Design review of the part built by this model. Coordinates are the model's own, in mm. A direction names the side the tool comes from. Round coordinates to 2 decimals unless told otherwise and drop trailing zeros. Loops run counter-clockwise (first coordinate to the right, second up) from the corner with the lowest first, then second, coordinate; pieces in that order, holes last. Notation, with made-up numbers: (82, 28) -> (99, 28) arc R24 cw to (99, 48) -> close; hole circle Ø4 at (16.5, 84.25). An arc over 180 degrees is marked (long way). Use a Markdown table: item, result. Add a question column.
from build123d import *

# Parameters (mm, degrees)
ESBO_O1_W                       = 143.01
ESBO_O1_H                       = 101.6
RESSALTO_EXTRUS_O1_DEPTH        = 6.35
ESBO_O2_R                       = 2
CORTE_EXTRUS_O1_DEPTH           = 13
ESBO_O3_R                       = 2.6
CORTE_EXTRUS_O2_DEPTH           = 7
ESBO_O4_R                       = 4
CORTE_EXTRUS_O3_DEPTH           = 0.55
CROQUIS1_R                      = 4
CORTAR_EXTRUIR1_DEPTH           = 2
CORTAR_EXTRUIR1_DRAFT           = -45
CORTAR_EXTRUIR1_PROFILE_2_DEPTH = 2
CORTAR_EXTRUIR1_PROFILE_2_DRAFT = -45
CORTAR_EXTRUIR1_PROFILE_3_DEPTH = 2
CORTAR_EXTRUIR1_PROFILE_3_DRAFT = -45
CORTAR_EXTRUIR1_PROFILE_4_DEPTH = 2
CORTAR_EXTRUIR1_PROFILE_4_DRAFT = -45
CORTAR_EXTRUIR1_PROFILE_5_DEPTH = 2
CORTAR_EXTRUIR1_PROFILE_5_DRAFT = -45
CORTAR_EXTRUIR1_PROFILE_6_DEPTH = 2
CORTAR_EXTRUIR1_PROFILE_6_DRAFT = -45
CORTAR_EXTRUIR1_PROFILE_7_DEPTH = 2
CORTAR_EXTRUIR1_PROFILE_7_DRAFT = -45
CORTAR_EXTRUIR1_PROFILE_8_DEPTH = 2
CORTAR_EXTRUIR1_PROFILE_8_DRAFT = -45


with BuildPart() as part:
    # Esboço1 → Ressalto-extrusão1 (new body)
    with BuildSketch(Plane.XY):
        Rectangle(ESBO_O1_W, ESBO_O1_H)
    extrude(amount=RESSALTO_EXTRUS_O1_DEPTH)

    # Esboço2 → Corte-extrusão1 (cut)
    with BuildSketch(Plane(origin=(0, 0, 0), x_dir=(-1, 0, 0), z_dir=(0, 0, -1))):
        with Locations((56.505, 47.125)):
            Circle(ESBO_O2_R)
        with Locations((26.505, 47.125)):
            Circle(ESBO_O2_R)
        with Locations((26.505, -47.125)):
            Circle(ESBO_O2_R)
        with Locations((56.505, -47.125)):
            Circle(ESBO_O2_R)
        with Locations((-26.505, 47.125)):
            Circle(ESBO_O2_R)
        with Locations((-56.505, 47.125)):
            Circle(ESBO_O2_R)
        with Locations((-56.505, -47.125)):
            Circle(ESBO_O2_R)
        with Locations((-26.505, -47.125)):
            Circle(ESBO_O2_R)
    extrude(amount=-CORTE_EXTRUS_O1_DEPTH, mode=Mode.SUBTRACT)

    # Esboço3 → Corte-extrusão2 (cut)
    with BuildSketch(Plane.XY.offset(6.35)):
        with Locations((20.8, -30.8)):
            Circle(ESBO_O3_R)
        with Locations((0, -30.8)):
            Circle(ESBO_O3_R)
        with Locations((-20.8, -30.8)):
            Circle(ESBO_O3_R)
        with Locations((-20.8, 24.2)):
            Circle(ESBO_O3_R)
        with Locations((0, 24.2)):
            Circle(ESBO_O3_R)
        with Locations((20.8, 24.2)):
            Circle(ESBO_O3_R)
    extrude(amount=-CORTE_EXTRUS_O2_DEPTH, mode=Mode.SUBTRACT)

    # Esboço4 → Corte-extrusão3 (cut)
    with BuildSketch(Plane(origin=(0, 0, 0), x_dir=(-1, 0, 0), z_dir=(0, 0, -1))):
        with Locations((-26.505, 47.125)):
            Circle(ESBO_O4_R)
        with Locations((-56.505, 47.125)):
            Circle(ESBO_O4_R)
        with Locations((-56.505, -47.125)):
            Circle(ESBO_O4_R)
        with Locations((-26.505, -47.125)):
            Circle(ESBO_O4_R)
        with Locations((26.505, -47.125)):
            Circle(ESBO_O4_R)
        with Locations((56.505, 47.125)):
            Circle(ESBO_O4_R)
        with Locations((26.505, 47.125)):
            Circle(ESBO_O4_R)
        with Locations((56.505, -47.125)):
            Circle(ESBO_O4_R)
    extrude(amount=-CORTE_EXTRUS_O3_DEPTH, mode=Mode.SUBTRACT)


with BuildPart() as cortar_extruir1_tool:
    # Croquis1 → Cortar-Extruir1 (with draft: the straight prism first)
    with BuildSketch(Plane(origin=(0, 0, 0.55), x_dir=(-1, 0, 0), z_dir=(0, 0, -1))):
        with Locations((56.505, 47.125)):
            Circle(CROQUIS1_R)
    extrude(amount=-CORTAR_EXTRUIR1_DEPTH)
    # Cortar-Extruir1: the draft: its side faces are tilted about the plane it starts from
    cortar_extruir1_sides = [cortar_extruir1_tool.faces().sort_by_distance(p)[0] for p in [
        (-52.505, 47.125, 1.55),
    ]]
    draft(cortar_extruir1_sides, Plane(origin=(0, 0, 0.55), x_dir=(-1, 0, 0), z_dir=(0, 0, -1)), CORTAR_EXTRUIR1_DRAFT)


with BuildPart() as part_1:
    add(part.part)

    # Cortar-Extruir1: cut by cortar_extruir1_tool
    add(cortar_extruir1_tool.part, mode=Mode.SUBTRACT)


with BuildPart() as cortar_extruir1_profile_2_tool:
    # Croquis1 → Cortar-Extruir1 profile 2 (with draft: the straight prism first)
    with BuildSketch(Plane(origin=(0, 0, 0.55), x_dir=(-1, 0, 0), z_dir=(0, 0, -1))):
        with Locations((26.505, 47.125)):
            Circle(CROQUIS1_R)
    extrude(amount=-CORTAR_EXTRUIR1_PROFILE_2_DEPTH)
    # Cortar-Extruir1 profile 2: the draft: its side faces are tilted about the plane it starts from
    cortar_extruir1_profile_2_sides = [cortar_extruir1_profile_2_tool.faces().sort_by_distance(p)[0] for p in [
        (-22.505, 47.125, 1.55),
    ]]
    draft(cortar_extruir1_profile_2_sides, Plane(origin=(0, 0, 0.55), x_dir=(-1, 0, 0), z_dir=(0, 0, -1)), CORTAR_EXTRUIR1_PROFILE_2_DRAFT)


with BuildPart() as part_2:
    add(part_1.part)

    # Cortar-Extruir1 profile 2: cut by cortar_extruir1_profile_2_tool
    add(cortar_extruir1_profile_2_tool.part, mode=Mode.SUBTRACT)


with BuildPart() as cortar_extruir1_profile_3_tool:
    # Croquis1 → Cortar-Extruir1 profile 3 (with draft: the straight prism first)
    with BuildSketch(Plane(origin=(0, 0, 0.55), x_dir=(-1, 0, 0), z_dir=(0, 0, -1))):
        with Locations((-26.505, 47.125)):
            Circle(CROQUIS1_R)
    extrude(amount=-CORTAR_EXTRUIR1_PROFILE_3_DEPTH)
    # Cortar-Extruir1 profile 3: the draft: its side faces are tilted about the plane it starts from
    cortar_extruir1_profile_3_sides = [cortar_extruir1_profile_3_tool.faces().sort_by_distance(p)[0] for p in [
        (30.505, 47.125, 1.55),
    ]]
    draft(cortar_extruir1_profile_3_sides, Plane(origin=(0, 0, 0.55), x_dir=(-1, 0, 0), z_dir=(0, 0, -1)), CORTAR_EXTRUIR1_PROFILE_3_DRAFT)


with BuildPart() as part_3:
    add(part_2.part)

    # Cortar-Extruir1 profile 3: cut by cortar_extruir1_profile_3_tool
    add(cortar_extruir1_profile_3_tool.part, mode=Mode.SUBTRACT)


with BuildPart() as cortar_extruir1_profile_4_tool:
    # Croquis1 → Cortar-Extruir1 profile 4 (with draft: the straight prism first)
    with BuildSketch(Plane(origin=(0, 0, 0.55), x_dir=(-1, 0, 0), z_dir=(0, 0, -1))):
        with Locations((-56.505, 47.125)):
            Circle(CROQUIS1_R)
    extrude(amount=-CORTAR_EXTRUIR1_PROFILE_4_DEPTH)
    # Cortar-Extruir1 profile 4: the draft: its side faces are tilted about the plane it starts from
    cortar_extruir1_profile_4_sides = [cortar_extruir1_profile_4_tool.faces().sort_by_distance(p)[0] for p in [
        (60.505, 47.125, 1.55),
    ]]
    draft(cortar_extruir1_profile_4_sides, Plane(origin=(0, 0, 0.55), x_dir=(-1, 0, 0), z_dir=(0, 0, -1)), CORTAR_EXTRUIR1_PROFILE_4_DRAFT)


with BuildPart() as part_4:
    add(part_3.part)

    # Cortar-Extruir1 profile 4: cut by cortar_extruir1_profile_4_tool
    add(cortar_extruir1_profile_4_tool.part, mode=Mode.SUBTRACT)


with BuildPart() as cortar_extruir1_profile_5_tool:
    # Croquis1 → Cortar-Extruir1 profile 5 (with draft: the straight prism first)
    with BuildSketch(Plane(origin=(0, 0, 0.55), x_dir=(-1, 0, 0), z_dir=(0, 0, -1))):
        with Locations((-56.505, -47.125)):
            Circle(CROQUIS1_R)
    extrude(amount=-CORTAR_EXTRUIR1_PROFILE_5_DEPTH)
    # Cortar-Extruir1 profile 5: the draft: its side faces are tilted about the plane it starts from
    cortar_extruir1_profile_5_sides = [cortar_extruir1_profile_5_tool.faces().sort_by_distance(p)[0] for p in [
        (60.505, -47.125, 1.55),
    ]]
    draft(cortar_extruir1_profile_5_sides, Plane(origin=(0, 0, 0.55), x_dir=(-1, 0, 0), z_dir=(0, 0, -1)), CORTAR_EXTRUIR1_PROFILE_5_DRAFT)


with BuildPart() as part_5:
    add(part_4.part)

    # Cortar-Extruir1 profile 5: cut by cortar_extruir1_profile_5_tool
    add(cortar_extruir1_profile_5_tool.part, mode=Mode.SUBTRACT)


with BuildPart() as cortar_extruir1_profile_6_tool:
    # Croquis1 → Cortar-Extruir1 profile 6 (with draft: the straight prism first)
    with BuildSketch(Plane(origin=(0, 0, 0.55), x_dir=(-1, 0, 0), z_dir=(0, 0, -1))):
        with Locations((-26.505, -47.125)):
            Circle(CROQUIS1_R)
    extrude(amount=-CORTAR_EXTRUIR1_PROFILE_6_DEPTH)
    # Cortar-Extruir1 profile 6: the draft: its side faces are tilted about the plane it starts from
    cortar_extruir1_profile_6_sides = [cortar_extruir1_profile_6_tool.faces().sort_by_distance(p)[0] for p in [
        (30.505, -47.125, 1.55),
    ]]
    draft(cortar_extruir1_profile_6_sides, Plane(origin=(0, 0, 0.55), x_dir=(-1, 0, 0), z_dir=(0, 0, -1)), CORTAR_EXTRUIR1_PROFILE_6_DRAFT)


with BuildPart() as part_6:
    add(part_5.part)

    # Cortar-Extruir1 profile 6: cut by cortar_extruir1_profile_6_tool
    add(cortar_extruir1_profile_6_tool.part, mode=Mode.SUBTRACT)


with BuildPart() as cortar_extruir1_profile_7_tool:
    # Croquis1 → Cortar-Extruir1 profile 7 (with draft: the straight prism first)
    with BuildSketch(Plane(origin=(0, 0, 0.55), x_dir=(-1, 0, 0), z_dir=(0, 0, -1))):
        with Locations((26.505, -47.125)):
            Circle(CROQUIS1_R)
    extrude(amount=-CORTAR_EXTRUIR1_PROFILE_7_DEPTH)
    # Cortar-Extruir1 profile 7: the draft: its side faces are tilted about the plane it starts from
    cortar_extruir1_profile_7_sides = [cortar_extruir1_profile_7_tool.faces().sort_by_distance(p)[0] for p in [
        (-22.505, -47.125, 1.55),
    ]]
    draft(cortar_extruir1_profile_7_sides, Plane(origin=(0, 0, 0.55), x_dir=(-1, 0, 0), z_dir=(0, 0, -1)), CORTAR_EXTRUIR1_PROFILE_7_DRAFT)


with BuildPart() as part_7:
    add(part_6.part)

    # Cortar-Extruir1 profile 7: cut by cortar_extruir1_profile_7_tool
    add(cortar_extruir1_profile_7_tool.part, mode=Mode.SUBTRACT)


with BuildPart() as cortar_extruir1_profile_8_tool:
    # Croquis1 → Cortar-Extruir1 profile 8 (with draft: the straight prism first)
    with BuildSketch(Plane(origin=(0, 0, 0.55), x_dir=(-1, 0, 0), z_dir=(0, 0, -1))):
        with Locations((56.505, -47.125)):
            Circle(CROQUIS1_R)
    extrude(amount=-CORTAR_EXTRUIR1_PROFILE_8_DEPTH)
    # Cortar-Extruir1 profile 8: the draft: its side faces are tilted about the plane it starts from
    cortar_extruir1_profile_8_sides = [cortar_extruir1_profile_8_tool.faces().sort_by_distance(p)[0] for p in [
        (-52.505, -47.125, 1.55),
    ]]
    draft(cortar_extruir1_profile_8_sides, Plane(origin=(0, 0, 0.55), x_dir=(-1, 0, 0), z_dir=(0, 0, -1)), CORTAR_EXTRUIR1_PROFILE_8_DRAFT)


with BuildPart() as part_8:
    add(part_7.part)

    # Cortar-Extruir1 profile 8: cut by cortar_extruir1_profile_8_tool
    add(cortar_extruir1_profile_8_tool.part, mode=Mode.SUBTRACT)


solid = part_8.part
1. Consider section B-B on x = 0. State the section outline as (y, z) points, plus the area to 3 significant figures.
2. Mouldability with a two-part tool opening along Y and no side actions: class faces 3 (the face through (-1, 1, 0)), 4 (the face through (-19.6, 21.893, 3.219)) as +Y half, -Y half, draft (parallel to the pull), parting line (faces both ways), or undercut.
3. Insertion check: P1, Ø7, axis at x = 56.505, y = -47.125, coming from the -Z side; P2, Ø5, axis at x = 26.505, y = 47.125, coming from the -Z side. Each pin has a flat end and moves straight along its axis. Give the tip position at first contact, or say it passes through.
4. To check wall thickness, follow probe 1 along Y at (x, z) = (20.8, 3.5); probe 2 along Y at (x, z) = (-22, 5.5); probe 3 along X at (y, z) = (23, 3.75) (3 decimals). State the ranges of each line that lie inside material, in increasing order. Write a range as from..to.
5. For faces 1 (the face through (-26.071, -49.077, 4.423)), 2 (the face through (-56.66, -43.13, 0.27)), list the 3-axis set-ups (+Z, -Z, +X, -X, +Y, -Y) from which the entire face can be reached by the end or side of a thin tool; tool diameter is ignored.
6. Consider section A-A on y = 24.2. State the section outline as (x, z) points (3 decimals).
7. Consider section C-C on z = 5. Give the number of separate pieces and of enclosed holes in the cut face, plus the area to 3 significant figures.
Verdict:
| question | item | result |
|---|---|---|
| 1 | outline | (-50.8, 0) -> (-33.4, 0) -> (-33.4, 6.35) -> (-50.8, 6.35) -> close; (-28.2, 0) -> (21.6, 0) -> (21.6, 6.35) -> (-28.2, 6.35) -> close; (26.8, 0) -> (50.8, 0) -> (50.8, 6.35) -> (26.8, 6.35) -> close |
| 1 | area | 579 mm² |
| 2 | face 3 | draft |
| 2 | face 4 | undercut |
| 3 | P1 | stops at z = 1.05 |
| 3 | P2 | stops at z = 2.05 |
| 4 | probe 1 | y = -50.8..-33.4, -28.2..21.6, 26.8..50.8 |
| 4 | probe 2 | y = -50.8..-33.11, -28.49..21.89, 26.51..50.8 |
| 4 | probe 3 | x = -71.505..-23.107, -18.493..-2.307, 2.307..18.493, 23.107..71.505 |
| 5 | face 1 | +Z, -Z |
| 5 | face 2 | -Z |
| 6 | outline | (-71.505, 0) -> (-23.4, 0) -> (-23.4, 6.35) -> (-71.505, 6.35) -> close; (-18.2, 0) -> (-2.6, 0) -> (-2.6, 6.35) -> (-18.2, 6.35) -> close; (2.6, 0) -> (18.2, 0) -> (18.2, 6.35) -> (2.6, 6.35) -> close; (23.4, 0) -> (71.505, 0) -> (71.505, 6.35) -> (23.4, 6.35) -> close |
| 7 | separate pieces | 1 |
| 7 | enclosed holes | 14 |
| 7 | area | 14,300 mm² |
